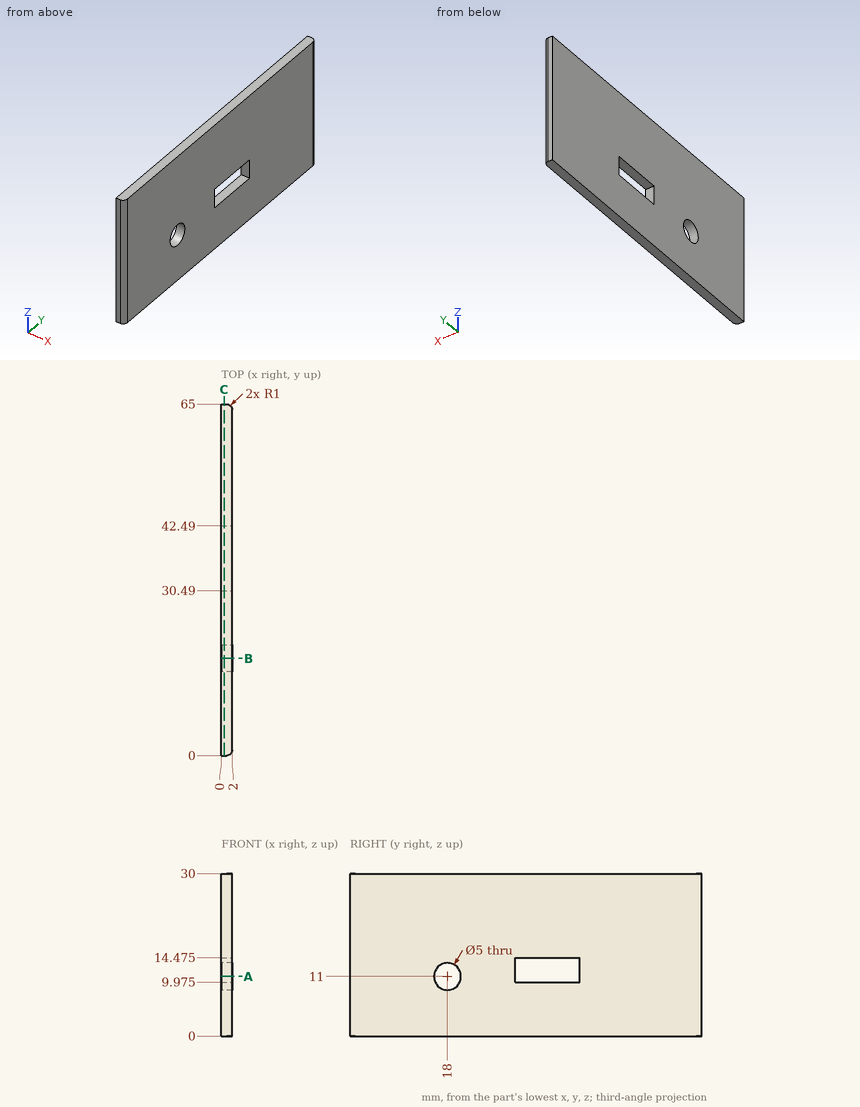
Design review of the part shown in the three views and the two pictorial views. Dimensions are in mm from the part's minimum x, y and z. Round coordinates to 2 decimals unless told otherwise and drop trailing zeros. Write each loop counter-clockwise with the first axis right and the second up, starting at its lowest first coordinate (ties: lowest second). Pieces come first, ordered by that corner, then holes. Notation, with made-up numbers: (3.25, -38.5) -> (26.25, -38.5) arc R23 cw to (26.25, -27.5) -> close; hole circle Ø4 at (80.25, 65.5). An arc over 180 degrees is marked (long way). Answer as a JSON object with one key per item and string values.
1. We need section A-A on z = 11. State the section outline as (x, y) points.
Results found:
{"outline": "(0, 0) -> (1, 0) arc R1 ccw to (2, 1) -> (2, 15.5) -> (0, 15.5) -> close; (0, 20.5) -> (2, 20.5) -> (2, 30.49) -> (0, 30.49) -> close; (0, 42.49) -> (2, 42.49) -> (2, 64) arc R1 ccw to (1, 65) -> (0, 65) -> close"}
2. We need section B-B on y = 18. State the section outline as (x, z) points, and give its area (3 significant figures).
Results found:
{"outline": "(0, 0) -> (2, 0) -> (2, 8.5) -> (0, 8.5) -> close; (0, 13.5) -> (2, 13.5) -> (2, 30) -> (0, 30) -> close", "area": "50.0 mm^2"}
3. We need section C-C on x = 0.55. State the section outline as (y, z) points (1 decimal), and give its area (3 significant figures).
Results found:
{"outline": "(0, 0) -> (65, 0) -> (65, 30) -> (0, 30) -> close; hole circle Ø5 at (18, 11); hole (30.5, 10) -> (42.5, 10) -> (42.5, 14.5) -> (30.5, 14.5) -> close", "area": "1,880 mm^2"}
4. To check wall thickness, follow line 1 along Z through (x, y) = (1.05, 38) (1 decimal); line 2 along Z through (x, y) = (1.45, 18); line 3 along Y through (x, z) = (0.85, 11.75) (1 decimal). State the ranges of each line that lie inside material, in increasing order.
Results found:
{"line 1": "z = 0 to 10, 14.5 to 30", "line 2": "z = 0 to 8.5, 13.5 to 30", "line 3": "y = 0 to 15.6, 20.4 to 30.5, 42.5 to 65"}
